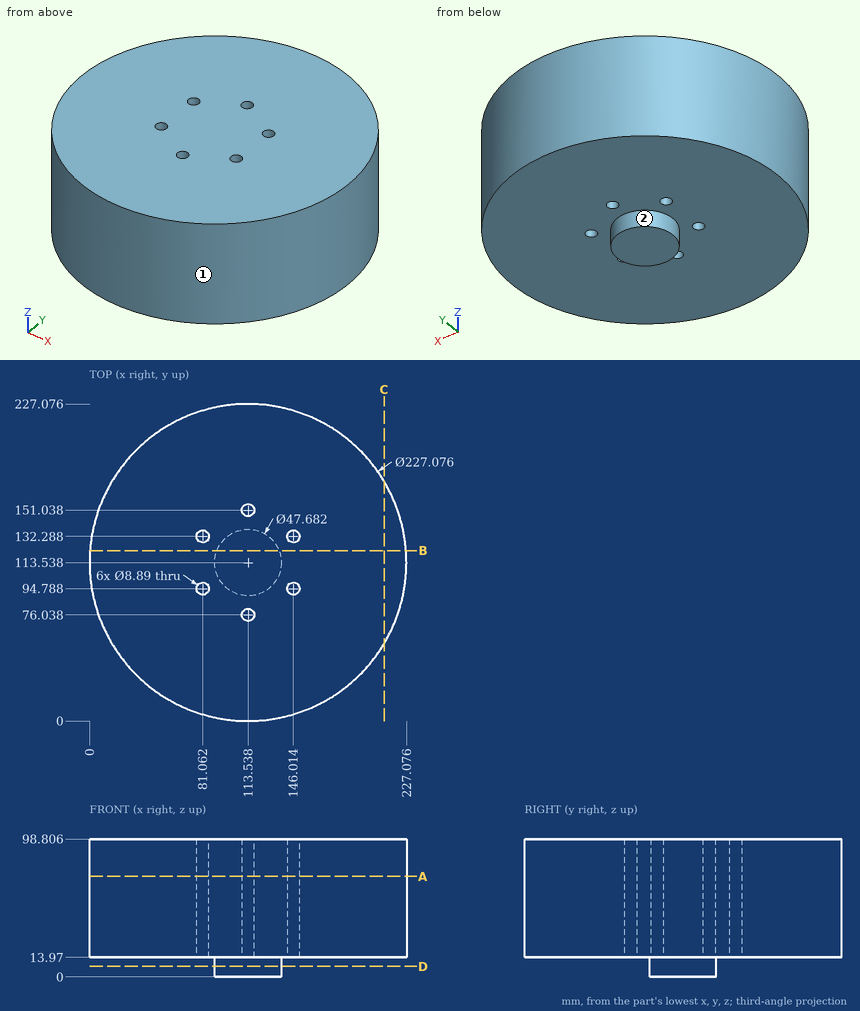
Print and shaded views of the part. All mm, measured from the part's lowest x, y and z. A direction names the side the tool comes from. Round coordinates to 2 decimals unless told otherwise and drop trailing zeros. Loops run counter-clockwise (first coordinate to the right, second up) from the corner with the lowest first, then second, coordinate; pieces in that order, holes last. Notation, with made-up numbers: (1.25, 47.5) -> (40.25, 47.5) arc R27 cw to (40.25, 71.5) -> close; hole circle Ø8 at (66, -11.5). An arc over 180 degrees is marked (long way). Use CSV: the item, a comma, the result in double quotes. Start each with the question number.
1) Cut at D-D, the plane z = 7.5. Write the cut outline in (x, y).
2) Which spindle directions (+Z, -Z, +X, -X, +Y, -Y) get a long thin tool onto all of the face, cutting with end or side? Do the marked faces 1 and 2. Say none if no direction does.
3) Cut at C-C, the plane x = 211. Write the cut outline in (y, z).
4) Cut at B-B, the plane y = 122. Write the cut outline in (x, z), plus the area to 3 significant figures.
5) Cut at A-A, the plane z = 72. Write the cut outline in (x, y) (1 decimal).
6) Drop flat-ended pins along their axis: P1, Ø2, axis at y = 136.5, z = 23.5, coming from the -X side; P2, Ø5, axis at y = 45, z = 45.5, coming from the +X side (1 decimal); P3, Ø5, axis at x = 173, y = 135.5, coming from the -Z side. Give the stop position or say it passes through.
7) Wall check: L1, parallel to Y at x = 84, z = 57.5 (1 decimal); L2, parallel to Z at x = 48, y = 182; L3, parallel to X at y = 111, z = 67. Give the ranges that are in metal, low to high. Write a range as [from, to].
Determined:
1,outline,"circle Ø47.68 at (113.54, 113.54)"
2,face 1,"+Z, -Z"
2,face 2,"-Z"
3,outline,"(55.3, 13.97) -> (171.78, 13.97) -> (171.78, 98.81) -> (55.3, 98.81) -> close"
4,outline,"(0.32, 13.97) -> (91.25, 13.97) -> (91.25, 0) -> (135.83, 0) -> (135.83, 13.97) -> (226.76, 13.97) -> (226.76, 98.81) -> (0.32, 98.81) -> close"
4,area,"19,800 mm2"
5,outline,"circle Ø227.1 at (113.5, 113.5); hole circle Ø8.9 at (81.1, 94.8); hole circle Ø8.9 at (81.1, 132.3); hole circle Ø8.9 at (113.5, 76); hole circle Ø8.9 at (113.5, 151); hole circle Ø8.9 at (146, 94.8); hole circle Ø8.9 at (146, 132.3)"
6,P1,"stops at x = 2.14"
6,P2,"stops at x = 205.9"
6,P3,"stops at z = 13.97"
7,L1,"y = [3.9, 91.5], [98.1, 129], [135.6, 223.2]"
7,L2,"z = [13.97, 98.81]"
7,L3,"x = [0.03, 227.05]"
